Check sheet for the modelled part. Datum: model origin and axes. Units: mm. Face numbers are marked on the shaded views. A direction names the side the tool comes from. Give positions to 0.01 mm unless a question says otherwise; leave off trailing zeros. Order: outer loops, then holes, each group sorted by start corner. A loop starts at its lowest first (then second) coordinate and runs counter-clockwise, first axis right, second up.
from build123d import *

# Parameters (mm, degrees)
ESQUISSE1_W             = 20
ESQUISSE1_H             = 14.3
BOSS_EXTRU_1_DEPTH      = 2
ESQUISSE2_W             = 20
ESQUISSE2_H             = 2
BOSS_EXTRU_2_DEPTH      = 20.55
ESQUISSE3_W             = 20
ESQUISSE3_H             = 2
BOSS_EXTRU_3_DEPTH      = 8
ESQUISSE4_R             = 1.5
ENL_V_MAT_EXTRU_2_DEPTH = 8
ESQUISSE5_R             = 1.5
ENL_V_MAT_EXTRU_3_DEPTH = 8


with BuildPart() as part:
    # Esquisse1 → Boss.-Extru.1 (new body)
    with BuildSketch(Plane.XY):
        with Locations((10, 7.15)):
            Rectangle(ESQUISSE1_W, ESQUISSE1_H)
    extrude(amount=BOSS_EXTRU_1_DEPTH)

    # Esquisse2 → Boss.-Extru.2 (add)
    with BuildSketch(Plane.XY.offset(2)):
        with Locations((10, 13.3)):
            Rectangle(ESQUISSE2_W, ESQUISSE2_H)
    extrude(amount=BOSS_EXTRU_2_DEPTH)

    # Esquisse3 → Boss.-Extru.3 (add)
    with BuildSketch(Plane(origin=(0, 14.3, 0), x_dir=(1, 0, 0), z_dir=(0, 1, 0))):
        with Locations((10, -21.55)):
            Rectangle(ESQUISSE3_W, ESQUISSE3_H)
    extrude(amount=BOSS_EXTRU_3_DEPTH)

    # Esquisse4 → Enlèv. mat.-Extru.2 (cut)
    with BuildSketch(Plane(origin=(0, 0, 0), x_dir=(-1, 0, 0), z_dir=(0, 0, -1))):
        with Locations((-17, 5.6)):
            Circle(ESQUISSE4_R)
        with Locations((-3, 5.6)):
            Circle(ESQUISSE4_R)
    extrude(amount=-ENL_V_MAT_EXTRU_2_DEPTH, mode=Mode.SUBTRACT)

    # Esquisse5 → Enlèv. mat.-Extru.3 (cut)
    with BuildSketch(Plane.XY.offset(22.55)):
        with Locations((13.91, 19.4)):
            Circle(ESQUISSE5_R)
    extrude(amount=-ENL_V_MAT_EXTRU_3_DEPTH, mode=Mode.SUBTRACT)


solid = part.part
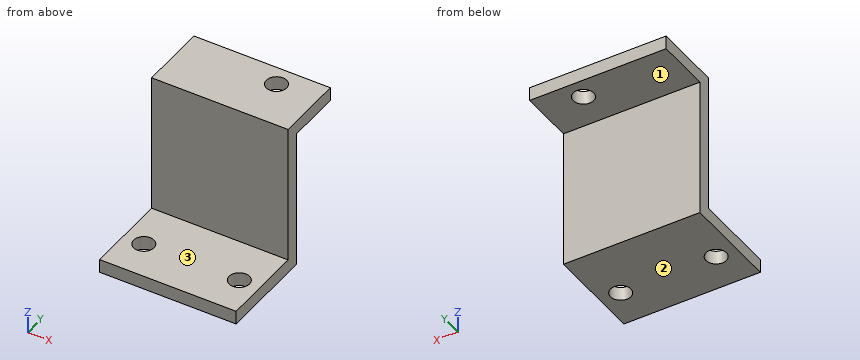
1) Section check A-A, the plane x = 13.91. Record the cut outline in (y, z).
Recorded:
outline: (0, 0) - (14.3, 0) - (14.3, 20.55) - (17.9, 20.55) - (17.9, 22.55) - (12.3, 22.55) - (12.3, 2) - (0, 2) - close; (20.9, 20.55) - (22.3, 20.55) - (22.3, 22.55) - (20.9, 22.55) - close
2) Set-up check for the marked faces 1, 2 and 3: record each of +Z, -Z, +X, -X, +Y, -Y from which the full face is reachable in a straight line by a thin tool's end or side.
Recorded:
face 1: -Z, +X, -X, +Y
face 2: -Z, +X, -X, +Y, -Y
face 3: +Z, +X, -X, -Y
3) Material ranges on L1, parallel to Y at x = 17, z = 1.2; L2, parallel to Y at x = 13.91, z = 21.35; L3, parallel to Y at x = 13.5, z = 18, recorded low to high.
Recorded:
L1: y = 0 to 4.1, 7.1 to 14.3
L2: y = 12.3 to 17.9, 20.9 to 22.3
L3: y = 12.3 to 14.3
4) Section check C-C, the plane y = 5.6. Record the cut outline in (x, z), then the cut area to 3 significant figures.
Recorded:
outline: (0, 0) - (1.5, 0) - (1.5, 2) - (0, 2) - close; (4.5, 0) - (15.5, 0) - (15.5, 2) - (4.5, 2) - close; (18.5, 0) - (20, 0) - (20, 2) - (18.5, 2) - close
area: 28.0 mm2
5) Depth check by flat-ended pin: pin 1 Ø6 at (x, z) = (9.5, 13.5) entering from +Y; pin 2 Ø3.5 at (x, y) = (11.5, 7.5) entering from +Z. Enter the tip coordinate at first touch or a pass-through.
Recorded:
pin 1: stops at y = 14.3
pin 2: stops at z = 2
6) Section check B-B, the plane y = 19.4. Record the cut outline in (x, z).
Recorded:
outline: (0, 20.55) - (12.41, 20.55) - (12.41, 22.55) - (0, 22.55) - close; (15.41, 20.55) - (20, 20.55) - (20, 22.55) - (15.41, 22.55) - close
7) Section check D-D, the plane x = 7.5. Record the cut outline in (y, z), then the cut area to 3 significant figures.
Recorded:
outline: (0, 0) - (14.3, 0) - (14.3, 20.55) - (22.3, 20.55) - (22.3, 22.55) - (12.3, 22.55) - (12.3, 2) - (0, 2) - close
area: 85.7 mm2
